Can you work these out from the model? Positions are in its coordinate system, mm. Face numbers are marked on the shaded views. A direction names the side the tool comes from. Give positions to 0.01 mm unless a question says otherwise; leave off trailing zeros. Order: outer loops, then holes, each group sorted by start corner. A loop starts at its lowest first (then second) coordinate and runs counter-clockwise, first axis right, second up. Notation, with made-up numbers: M 4.5,54.25 L 29.5,54.25 A29 ccw 29.5,82.25 Z; hole C 62,-0.5 d6. An arc over 180 degrees is marked long. Answer as a JSON object with one key per item and string values.
```python
from build123d import *

# Parameters (mm, degrees)
SKETCH_1_R          = 12.935
EXTRUDE_1_DEPTH     = 11
SKETCH_2_R          = 14.935
EXTRUDE_2_DEPTH     = 1
EXTRUDE_START       = 1
SKETCH_3_R          = 14.935
EXTRUDE_3_DEPTH     = 1
SKETCH_4_R          = 11
EXTRUDE_4_DEPTH     = 9
SKETCH_5_R          = 5
CUT_EXTRUDE_1_DEPTH = 30


with BuildPart() as part:
    # 草图1 → 凸台-拉伸1 (new body)
    with BuildSketch(Plane(origin=(0, 0, 0), x_dir=(0, 0, -1), z_dir=(1, 0, 0))):
        Circle(SKETCH_1_R)
    extrude(amount=EXTRUDE_1_DEPTH)

    # 草图2 → 凸台-拉伸2 (add)
    with BuildSketch(Plane(origin=(11, 0, 0), x_dir=(0, 0, -1), z_dir=(1, 0, 0))):
        Circle(SKETCH_2_R)
    extrude(amount=EXTRUDE_2_DEPTH)

    # 草图3 → 凸台-拉伸3 (add)
    with BuildSketch(Plane.ZY.offset(EXTRUDE_START)):
        with Locations(Location((0, 0, 0), (0, 0, 180))):
            Circle(SKETCH_3_R)
    extrude(amount=-EXTRUDE_3_DEPTH)

    # 草图4 → 凸台-拉伸4 (add)
    with BuildSketch(Plane.ZY.offset(1)):
        with Locations(Location((0, 0, 0), (0, 0, 180))):
            Circle(SKETCH_4_R)
    extrude(amount=EXTRUDE_4_DEPTH)

    # 草图5 → 切除-拉伸1 (cut)
    with BuildSketch(Plane.ZY.offset(10)):
        Circle(SKETCH_5_R)
    extrude(amount=-CUT_EXTRUDE_1_DEPTH, mode=Mode.SUBTRACT)


solid = part.part
```
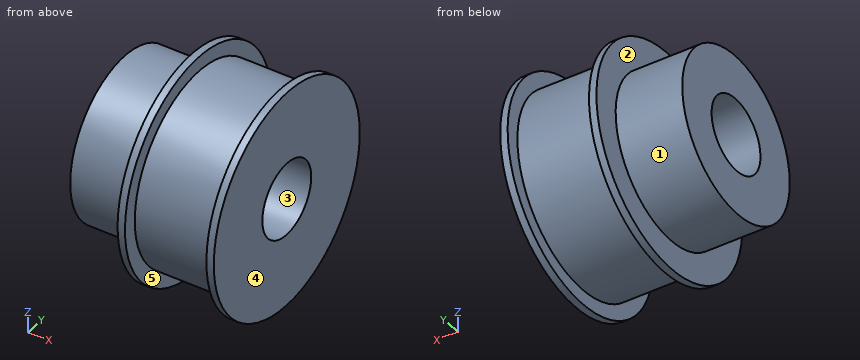
1) I'm going to push flat-ended pins straight in: pin 1 Ø3 at (x, z) = (7, -4.5) entering from -Y; pin 2 Ø10 at (x, y) = (7, 4) entering from -Z; pin 3 Ø9 at (y, z) = (-1.5, 0.5) entering from -X; pin 4 Ø2 at (x, z) = (9.5, 7.5) entering from +Y. Where does each tip first touch, or does it pass through?
Results found:
{"pin 1": "stops at y = -12.58", "pin 2": "stops at z = -14.9", "pin 3": "stops at x = -10", "pin 4": "stops at y = 11.18"}
2) I want a section at C-C on x = 7.25. Write out the boundary of the cut face in (y, z) (3 decimals).
Results found:
{"outline": "C 0,0 d25.87; hole C 0,0 d10"}
3) Thinking about a two-plate mould opening in Z: for the marked faces 1, 2 and 3, which applies, pulls with the +Z half, pulls with the -Z half, needs draft (parallel to the pull), parting line crosses it, or undercut?
Results found:
{"face 1": "parting line crosses it", "face 2": "needs draft", "face 3": "undercut"}
4) I want a section at D-D on z = -11.5. Write out the boundary of the cut face in (x, y), and give its area (3 significant figures).
Results found:
{"outline": "M -1,-9.53 L 0,-9.53 L 0,-5.92 L 11,-5.92 L 11,-9.53 L 12,-9.53 L 12,9.53 L 11,9.53 L 11,5.92 L 0,5.92 L 0,9.53 L -1,9.53 Z", "area": "168 mm²"}
5) For the marked faces 4 and 5, which set-ups out of +Z, -Z, +X, -X, +Y, -Y let a thin tool reach every point of the face, with its end or its side?
Results found:
{"face 4": "+Z, -Z, +X, +Y, -Y", "face 5": "none"}
6) I need wall thicknesses on L1, parallel to X at y = 9.75, z = -11; L2, parallel to Y at x = 5, z = 0 (3 decimals); L3, parallel to Y at x = -4.5, z = 3.25. Which ranges of each line are inside material? Lowest first, please.
Results found:
{"L1": "x = -1 to 0, 11 to 12", "L2": "y = -12.935 to -5, 5 to 12.935", "L3": "y = -10.51 to -3.8, 3.8 to 10.51"}
7) I want a section at A-A on y = 0. Write out the boundary of the cut face in (x, z) (3 decimals), and give its area (3 significant figures).
Results found:
{"outline": "M -10,-11 L -1,-11 L -1,-14.935 L 0,-14.935 L 0,-12.935 L 11,-12.935 L 11,-14.935 L 12,-14.935 L 12,-5 L -10,-5 Z; M -10,5 L 12,5 L 12,14.935 L 11,14.935 L 11,12.935 L 0,12.935 L 0,14.935 L -1,14.935 L -1,11 L -10,11 Z", "area": "322 mm²"}
